```python
from build123d import *

# Parameters (mm, degrees)
PAD005_DEPTH            = 4
SKETCH014_R             = 2.5
PAD006_DEPTH            = 2
CHAMFER_SIZE            = 0.25
BODY005_ROLL_ANGLE      = -150
BODY005_PLACEMENT_ANGLE = 180


with BuildPart() as part:
    # Sketch013 → Pad005 (new body, symmetric)
    with BuildSketch(Plane.YZ):
        with BuildLine():
            ThreePointArc((0, 3), (-3, 0), (0, -3))
            Line((0, 3), (0, -3))
        make_face()
    extrude(amount=PAD005_DEPTH, both=True)

    # Sketch014 (on Face2 of Pad005) → Pad006 (join)
    with BuildSketch(Plane.ZX):
        Circle(SKETCH014_R)
    extrude(amount=PAD006_DEPTH)

    # Chamfer
    chamfer_edges = [part.edges().sort_by_distance(p)[0] for p in [
        (0, 2, -2.5),
        (-4, -3, 0),
        (-4, 0, 0),
        (4, -3, 0),
        (4, 0, 0),
        (0, 0, -3),
        (0, 0, 3),
    ]]
    chamfer(chamfer_edges, length=CHAMFER_SIZE)


with BuildPart() as part_1:
    # Body005 roll: moved
    add(part.part.rotate(Axis((0, 0, 0), (1, 0, 0)), BODY005_ROLL_ANGLE))


with BuildPart() as part_2:
    # Body005 placement: moved
    add(part_1.part.moved(Location((0, 6.772758664, 16.05))).rotate(Axis((0, 6.772758664, 16.05), (0, 0, 1)), BODY005_PLACEMENT_ANGLE))


solid = part_2.part
```
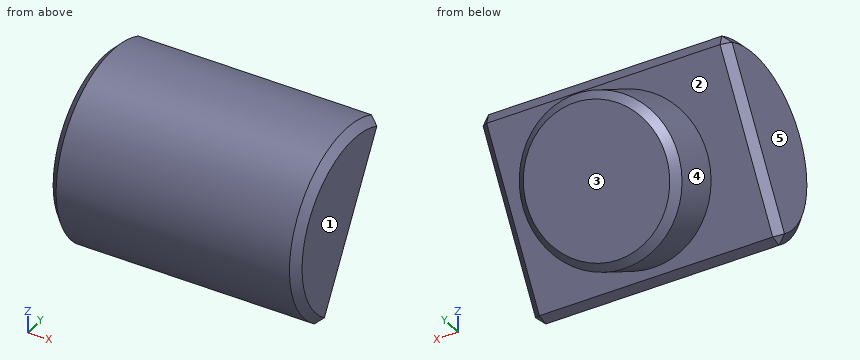
Can you work these out from the model? Positions are in its coordinate system, mm. Face numbers are marked on the shaded views. A direction names the side the tool comes from. Give positions to 0.01 mm unless a question says otherwise; leave off trailing zeros. Use a Markdown table: item, result. Add a question column.
Q1. If we mould it in two halves opening along Y, with no side actions, what happens to the marked faces 3, 4 and 5? For each: released by +Y, released by -Y, zero draft, split by the parting line, or undercut.
Q2. I'm going to push a flat-ended pin straight in: pin 1 (1 mm diameter, centred on x = 1, z = 15.5, fed in from +Y). Where does the tip first touch, or does it pass through?
Q3. Please list where these lines run through material, in increasing order: line 1 along X through (y, z) = (8.05, 15.25); line 2 along Z through (x, y) = (-2.75, 6.85); line 3 along Y through (x, z) = (-0.25, 17).
Q4. On a 3-axis mill with a long thin cutter (end or side, diameter ignored), from which of +Z, -Z, +X, -X, +Y, -Y can I reach the whole of each face in a straight line? I mean the marked faces 1 and 2. Say none if no direction works.
Answers follow:
| question | item | result |
|---|---|---|
| 1 | face 3 | released by +Y |
| 1 | face 4 | undercut |
| 1 | face 5 | zero draft |
| 2 | pin 1 | stops at y = 9.05 |
| 3 | line 1 | x = -2.5 to 2.5 |
| 3 | line 2 | z = 16.18 to 19.05 |
| 3 | line 3 | y = 3.93 to 9.62 |
| 4 | face 1 | +Z, -Z, +X, +Y, -Y |
| 4 | face 2 | none |
